The drawing under review shows one solid part. Ordinate dimensions are in mm from its lowest x, y, z. Give positions to 0.01 mm unless a question says otherwise; leave off trailing zeros. Write each loop counter-clockwise with the first axis right and the second up, starting at its lowest first coordinate (ties: lowest second). Pieces come first, ordered by that corner, then holes. Notation, with made-up numbers: (17, -18.5) -> (74, -18.5) arc R22 cw to (74, 17.5) -> close; hole circle Ø10 at (88, 12). An arc over 180 degrees is marked (long way). Write item = value, one per line.
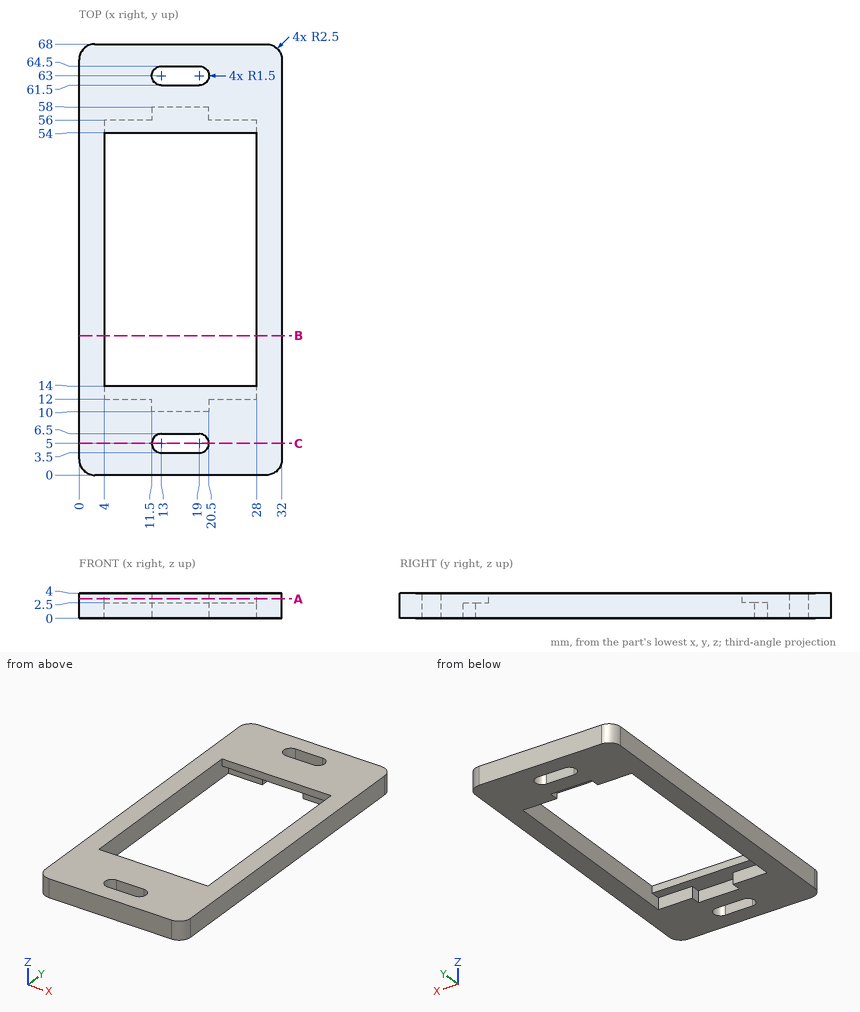
(1) For pin 1 (10 mm diameter, centred on x = 18.5, y = 50.5, fed in from -Z), flat-tipped, find the tip position at first contact; note if it passes through.
Answers below:
pin_1 = 2.5
(2) Take a section at C-C (y = 5). Write out the cut boundary in (x, z).
Answers below:
outline = (0, 0) -> (11.5, 0) -> (11.5, 4) -> (0, 4) -> close; (20.5, 0) -> (32, 0) -> (32, 4) -> (20.5, 4) -> close
(3) Take a section at A-A (z = 3.1). Write out the cut boundary in (x, y).
Answers below:
outline = (0, 2.5) arc R2.5 ccw to (2.5, 0) -> (29.5, 0) arc R2.5 ccw to (32, 2.5) -> (32, 65.5) arc R2.5 ccw to (29.5, 68) -> (2.5, 68) arc R2.5 ccw to (0, 65.5) -> close; hole (4, 14) -> (28, 14) -> (28, 54) -> (4, 54) -> close; hole (13, 3.5) -> (19, 3.5) arc R1.5 ccw to (19, 6.5) -> (13, 6.5) arc R1.5 ccw to start; hole (13, 61.5) -> (19, 61.5) arc R1.5 ccw to (19, 64.5) -> (13, 64.5) arc R1.5 ccw to start
(4) Take a section at B-B (y = 22). Write out the cut boundary in (x, z), plus the area to 3 significant figures.
Answers below:
outline = (0, 0) -> (4, 0) -> (4, 4) -> (0, 4) -> close; (28, 0) -> (32, 0) -> (32, 4) -> (28, 4) -> close
area = 32.0 mm^2
(5) To check wall thickness, follow probe 1 along Y at (x, z) = (13, 1.75); probe 2 along Y at (x, z) = (13, 3); probe 3 along X at (y, z) = (49, 3.15). State the ranges of each line that lie inside material, in increasing order.
Answers below:
probe_1 = 0 to 3.5, 6.5 to 10, 58 to 61.5, 64.5 to 68
probe_2 = 0 to 3.5, 6.5 to 14, 54 to 61.5, 64.5 to 68
probe_3 = 0 to 4, 28 to 32
